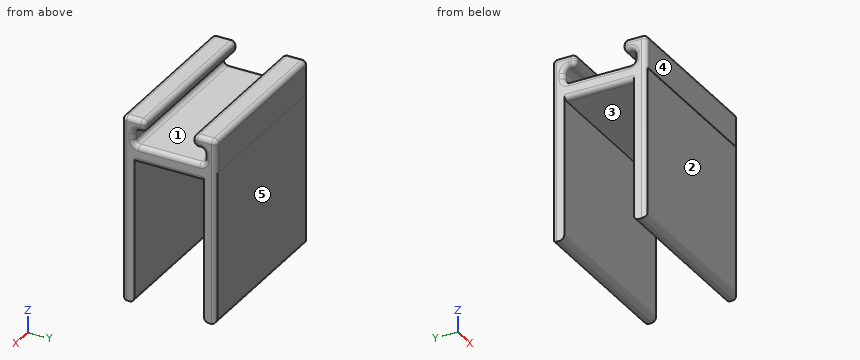
from build123d import *

# Parameters (mm, degrees)
F1_DEPTH = 44.45
F2_R     = 1.27


with BuildPart() as f1:
    # F0 (on Right) → F1 (new body)
    with BuildSketch(Plane.YZ):
        with BuildLine():
            Line((10.668, -24.967044556), (11.303, -24.967044556))
            ThreePointArc((11.303, -24.967044556), (12.2010256121, -24.5950701681), (12.573, -23.697044556))
            Line((12.573, -23.697044556), (12.573, 15.9512687449))
            Line((12.573, 15.9512687449), (12.7, 15.9512687449))
            Line((12.7, 15.9512687449), (12.7, 23.697044556))
            ThreePointArc((12.7, 23.697044556), (12.3280256121, 24.5950701681), (11.43, 24.967044556))
            Line((11.43, 24.967044556), (7.62, 24.967044556))
            ThreePointArc((7.62, 24.967044556), (6.7219743879, 24.5950701681), (6.35, 23.697044556))
            Line((6.35, 23.697044556), (6.35, 23.062044556))
            ThreePointArc((6.35, 23.062044556), (6.7219743879, 22.1640189439), (7.62, 21.792044556))
            Line((7.62, 21.792044556), (8.255, 21.792044556))
            ThreePointArc((8.255, 21.792044556), (9.1530256121, 21.4200701681), (9.525, 20.522044556))
            Line((9.525, 20.522044556), (9.525, 19.023438717))
            ThreePointArc((9.525, 19.023438717), (9.1530256121, 18.1254131049), (8.255, 17.753438717))
            Line((8.255, 17.753438717), (-8.255, 17.753438717))
            ThreePointArc((-8.255, 17.753438717), (-9.1530256121, 18.1254131049), (-9.525, 19.023438717))
            Line((-9.525, 19.023438717), (-9.525, 20.522044556))
            ThreePointArc((-9.525, 20.522044556), (-9.1530256121, 21.4200701681), (-8.255, 21.792044556))
            Line((-8.255, 21.792044556), (-7.62, 21.792044556))
            ThreePointArc((-7.62, 21.792044556), (-6.7219743879, 22.1640189439), (-6.35, 23.062044556))
            Line((-6.35, 23.062044556), (-6.35, 23.697044556))
            ThreePointArc((-6.35, 23.697044556), (-6.7219743879, 24.5950701681), (-7.62, 24.967044556))
            Line((-7.62, 24.967044556), (-11.43, 24.967044556))
            ThreePointArc((-11.43, 24.967044556), (-12.3280256121, 24.5950701681), (-12.7, 23.697044556))
            Line((-12.7, 23.697044556), (-12.7, 15.9512687449))
            Line((-12.7, 15.9512687449), (-12.573, 15.9512687449))
            Line((-12.573, 15.9512687449), (-12.573, -23.697044556))
            ThreePointArc((-12.573, -23.697044556), (-12.2010256121, -24.5950701681), (-11.303, -24.967044556))
            Line((-11.303, -24.967044556), (-10.668, -24.967044556))
            ThreePointArc((-10.668, -24.967044556), (-9.7699743879, -24.5950701681), (-9.398, -23.697044556))
            Line((-9.398, -23.697044556), (-9.398, 13.132955444))
            Line((-9.398, 13.132955444), (9.398, 13.132955444))
            Line((9.398, 13.132955444), (9.398, -23.697044556))
            ThreePointArc((9.398, -23.697044556), (9.7699743879, -24.5950701681), (10.668, -24.967044556))
        make_face()
    extrude(amount=F1_DEPTH)

    # F2
    f2_edges = [f1.edges().sort_by_distance(p)[0] for p in [
        (44.45, -12.7, 19.824157),
        (44.45, -9.525, 24.967045),
        (0, 0, 17.753439),
        (0, 0, 13.132955),
        (44.45, 0, 13.132955),
    ]]
    fillet(f2_edges, radius=F2_R)


solid = f1.part
For this review, take the finished solid that the model builds, in its own axes (mm). Face numbers are marked on the shaded views. A direction names the side the tool comes from. Coordinates: 2 decimals unless noted, no trailing zeros. Loops run counter-clockwise (first coordinate to the right, second up) from the corner with the lowest first, then second, coordinate; pieces in that order, holes last. Notation, with made-up numbers: (28.25, 86.5) - (84.25, 86.5) arc R15 ccw to (84.25, 101.5) - close; hole circle Ø1 at (-32.5, -39.75). An arc over 180 degrees is marked (long way). Use a Markdown table: item, result. Add a question column.
Item 1: We need section A-A (z = -3.5). Give the boundary of the cut face in (x, y).
Item 2: We need section C-C (y = 5.25). Give the boundary of the cut face in (x, z).
Item 3: For line 1 (Y direction, x = 10.5, z = 10.5); line 2 (Z direction, x = 30, y = -3.5); line 3 (X direction, y = -11.5, z = 13.5), list the stretches that pass through material, from the lowest coordinate up.
Item 4: Tool access review of the marked faces 1, 2, 3, 4 and 5: name each direction out of +Z, -Z, +X, -X, +Y, -Y from which nothing blocks a thin tool from reaching the whole face with its end or side.
Item 5: Insertion check: pin 1 Ø1.5 at (x, z) = (20, -1) entering from -Y; pin 2 Ø8.5 at (x, y) = (14.5, -1.5) entering from +Z; pin 3 Ø11.5 at (x, z) = (31.5, -10.5) entering from +Y. Each pin has a flat end and moves straight along its axis. Give the tip position at first contact, or say it passes through.
Results list:
| question | item | result |
|---|---|---|
| 1 | outline | (0, -11.43) arc R1.27 ccw to (0.72, -12.57) - (43.73, -12.57) arc R1.27 ccw to (44.45, -11.43) - (44.45, -9.4) - (0, -9.4) - close; (0, 9.4) - (44.45, 9.4) - (44.45, 11.43) arc R1.27 ccw to (43.73, 12.57) - (0.72, 12.57) arc R1.27 ccw to (0, 11.43) - close |
| 2 | outline | (0, 14.4) arc R1.27 ccw to (1.27, 13.13) - (43.18, 13.13) arc R1.27 ccw to (44.45, 14.4) - (44.45, 16.48) arc R1.27 ccw to (43.18, 17.75) - (1.27, 17.75) arc R1.27 ccw to (0, 16.48) - close |
| 3 | line 1 | y = -12.57 to -9.4, 9.4 to 12.57 |
| 3 | line 2 | z = 13.13 to 17.75 |
| 3 | line 3 | x = 0 to 44.45 |
| 4 | face 1 | +X, -X |
| 4 | face 2 | -Z, +X, -X, -Y |
| 4 | face 3 | -Z, +X, -X |
| 4 | face 4 | +Z, -Z, +X, -X, -Y |
| 4 | face 5 | -Z, +X, -X, +Y |
| 5 | pin 1 | stops at y = -12.57 |
| 5 | pin 2 | stops at z = 17.75 |
| 5 | pin 3 | stops at y = 12.57 |
